from build123d import *

# Parameters (mm, degrees)
REVOLVE8_ANGLE      = 22.5
BOSS_EXTRUDE3_START = 12.7
BOSS_EXTRUDE3_DEPTH = 12.7
BOSS_EXTRUDE4_DEPTH = 12.7
SKETCH12_R          = 1.905
CUT_EXTRUDE4_DEPTH  = 3.175
SKETCH13_R          = 1.905
CUT_EXTRUDE5_DEPTH  = 3.175


with BuildPart() as part:
    # Sketch9 → Revolve8 (revolve)
    with BuildSketch(Plane.XY):
        with BuildLine():
            Line((-49.2252, -98.425), (-52.4002, -98.425))
            Line((-52.4002, -98.425), (-52.4002, -150.8252))
            Line((-52.4002, -150.8252), (52.4002, -150.8252))
            Line((52.4002, -150.8252), (52.4002, -98.425))
            Line((52.4002, -98.425), (49.2252, -98.425))
            ThreePointArc((49.2252, -98.425), (0, -147.6502), (-49.2252, -98.425))
        make_face()
    revolve(axis=Axis((-38.048924234, 0, 0), (-1, 0, 0)), revolution_arc=REVOLVE8_ANGLE)

    # Sketch11 → Boss-Extrude3 (add)
    with BuildSketch(Plane.ZY.offset(52.4002).offset(BOSS_EXTRUDE3_START)):
        with BuildLine():
            Line((0, -98.425), (0, -150.8252))
            ThreePointArc((0, -150.8252), (1.5875, -150.816845209), (3.174824124, -150.791781762))
            Line((3.174824124, -150.791781762), (2.623242695, -98.390036197))
            ThreePointArc((2.623242695, -98.390036197), (1.311737846, -98.416258661), (0, -98.425))
        make_face()
    extrude(amount=-BOSS_EXTRUDE3_DEPTH)

    # Sketch10 → Boss-Extrude4 (add)
    with BuildSketch(Plane(origin=(52.4002, 0, 0), x_dir=(0, 0, -1), z_dir=(1, 0, 0))):
        with BuildLine():
            Line((0, -98.425), (0, -150.8252))
            Line((0, -150.8252), (-3.174824124, -150.791781762))
            Line((-3.174824124, -150.791781762), (-3.174824124, -98.37378267))
            ThreePointArc((-3.174824124, -98.37378267), (-1.587618613, -98.412194834), (0, -98.425))
        make_face()
    extrude(amount=BOSS_EXTRUDE4_DEPTH)

    # Sketch12 → Cut-Extrude4 (cut)
    with BuildSketch(Plane.XY.offset(3.174824124)):
        with Locations((60.550186424, -111.886000657)):
            Circle(SKETCH12_R)
        with Locations((60.550186424, -141.566764633)):
            Circle(SKETCH12_R)
        with Locations((60.550186424, -127.4445)):
            Circle(SKETCH12_R)
    extrude(amount=-CUT_EXTRUDE4_DEPTH, mode=Mode.SUBTRACT)

    # Sketch13 → Cut-Extrude5 (cut)
    with BuildSketch(Plane(origin=(0, -0.008353865, 1.587675876), x_dir=(1, 0, 0), z_dir=(-8.55203915581382e-15, 0.010525429437517081, 0.9999446061333377))):
        with Locations(Location((-60.754019077, -141.521938379, 0), (0, 0, 270))):
            Circle(SKETCH13_R)
        with Locations(Location((-60.754019077, -112.479497113, 0), (0, 0, 270))):
            Circle(SKETCH13_R)
        with Locations(Location((-60.754019077, -127.4445, 0), (0, 0, 270))):
            Circle(SKETCH13_R)
    extrude(amount=-CUT_EXTRUDE5_DEPTH, mode=Mode.SUBTRACT)


solid = part.part
Check sheet for the modelled part. Datum: model origin and axes. Units: mm. A direction names the side the tool comes from. Round coordinates to 2 decimals unless told otherwise and drop trailing zeros. Order: outer loops, then holes, each group sorted by start corner. A loop starts at its lowest first (then second) coordinate and runs counter-clockwise, first axis right, second up.
(1) Go/stop test with flat-tipped pins: P1, Ø6, axis at y = -123, z = 14, coming from the +X side; P2, Ø4.5, axis at x = 60.55, y = -111.89, coming from the +Z side; P3, Ø16.5, axis at y = -108.5, z = 20.5, coming from the -X side. Record where each tip stops, or that it passes through.
(2) Cross-section at B-B, the plane x = -17. Enter the section's corners in (y, z), and give its area (3 significant figures).
(3) Draft check along Y on faces 1 (the cylindrical face through (58.647, -141.483, 1.61)), 2 (the flat face through (59, -125, 3.175)), 3 (the flat face through (-8.008, -136.542, 56.557)). Enter one of: pulls with the +Y half, pulls with the -Y half, needs draft (parallel to the pull), parting line crosses it, or undercut.
(4) Scan lines: probe 1 along X at (y, z) = (-101.5, 13.5); probe 2 along Z at (x, y) = (-57, -137.5); probe 3 along Y at (x, z) = (-1.5, 36). Record each from-to range of solid material in increasing order.
(5) Cross-section at A-A, the plane x = 56.5. Enter the section's corners in (y, z) (3 decimals), and give its area (3 significant figures).
(6) Access from +Z, -Z, +X, -X, +Y, -Y to the whole of each face (thin tool, end or side, straight path). Record for faces 4 (the cylindrical face through (58.647, -127.361, 1.61)), 5 (the flat face through (52.4, -120, 25)).
Check sheet entries:
1. P1: stops at x = 52.4
1. P2: stops at z = 3.17
1. P3: stops at x = -52.4
2. outline: (-150.83, 0) - (-144.62, 0) arc R144.62 cw to (-133.61, 55.34) - (-139.34, 57.72) arc R150.83 ccw to start
2. area: 360 mm2
3. face 1: undercut
3. face 2: needs draft
3. face 3: pulls with the +Y half
4. probe 1: x = -52.4 to -49.06, 49.06 to 52.4
4. probe 2: z = 0 to 3.03
4. probe 3: y = -146.47 to -143.17
5. outline: (-150.825, 0) - (-98.425, 0) arc R98.425 cw to (-98.374, 3.175) - (-150.792, 3.175) - close
5. area: 166 mm2
6. face 4: +Z, -Z
6. face 5: +Z, +X, +Y, -Y
